Verification items for this drawing (mm, ordinates from the low corner). A direction names the side the tool comes from. Round coordinates to 2 decimals unless told otherwise and drop trailing zeros. Write each loop counter-clockwise with the first axis right and the second up, starting at its lowest first coordinate (ties: lowest second). Pieces come first, ordered by that corner, then holes.
Item 1: Cross-section at D-D (y = 16.5). Enter the section's corners in (x, z).
Item 2: Cross-section at A-A (z = 63.5). Enter the section's corners in (x, y), then the cut area to 3 significant figures.
Item 3: Access from +Z, -Z, +X, -X, +Y, -Y to the whole of each face (thin tool, end or side, straight path). Record for the marked faces 1, 2 and 3.
Item 4: Depth check by flat-ended pin: P1, Ø12.5, axis at x = 110.5, z = 24, coming from the -Y side; P2, Ø15, axis at y = 104.775, z = 22.225, coming from the +X side; P3, Ø6, axis at x = 109, z = 22.5, coming from the +Y side. Enter the tip coordinate at first touch or a pass-through.
Item 5: Draft check along X on the marked faces 4, 5 and 6. Enter one of: pulls with the +X half, pulls with the -X half, needs draft (parallel to the pull), parting line crosses it, or undercut.
Item 6: Scan lines: probe 1 along X at (y, z) = (63.5, 3.75) (3 decimals); probe 2 along Z at (x, y) = (63.5, 2.5); probe 3 along Z at (x, y) = (61.5, 70). Record each from-to range of solid material in increasing order.
Item 7: Cross-section at C-C (y = 63.5). Enter the section's corners in (x, z) (3 decimals), then the cut area to 3 significant figures.
Item 8: Cross-section at B-B (x = 63.5). Enter the section's corners in (y, z), then the cut area to 3 significant figures.
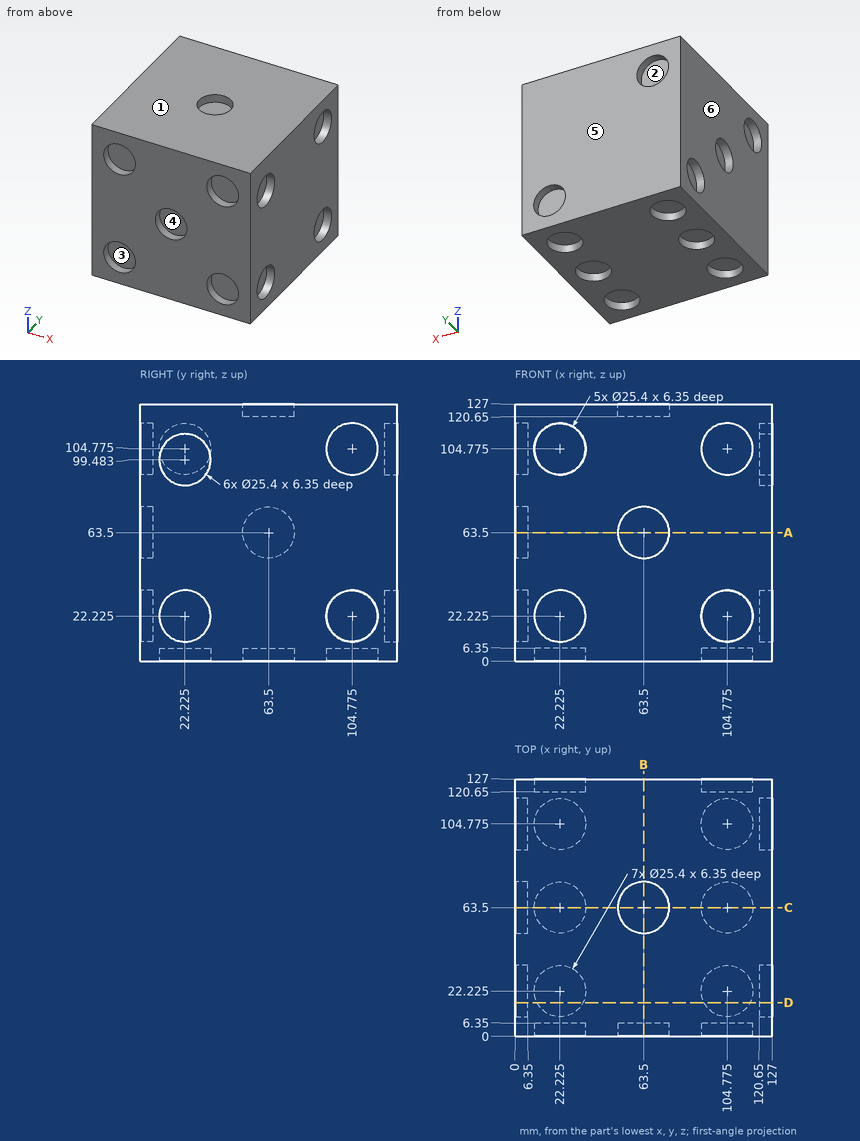
Resolved:
1. outline: (0, 0) - (10.89, 0) - (10.89, 6.35) - (33.56, 6.35) - (33.56, 0) - (93.44, 0) - (93.44, 6.35) - (116.11, 6.35) - (116.11, 0) - (127, 0) - (127, 10.89) - (120.65, 10.89) - (120.65, 33.56) - (127, 33.56) - (127, 88.15) - (120.65, 88.15) - (120.65, 110.82) - (127, 110.82) - (127, 127) - (0, 127) - (0, 116.11) - (6.35, 116.11) - (6.35, 93.44) - (0, 93.44) - close
2. outline: (0, 0) - (50.8, 0) - (50.8, 6.35) - (76.2, 6.35) - (76.2, 0) - (127, 0) - (127, 127) - (0, 127) - (0, 76.2) - (6.35, 76.2) - (6.35, 50.8) - (0, 50.8) - close
2. area: 15,800 mm2
3. face 1: +Z, +X, -X, +Y, -Y
3. face 2: +Y
3. face 3: -Y
4. P1: stops at y = 6.35
4. P2: stops at x = 120.65
4. P3: stops at y = 120.65
5. face 4: undercut
5. face 5: needs draft
5. face 6: pulls with the -X half
6. probe 1: x = 0 to 9.525, 34.925 to 92.075, 117.475 to 127
6. probe 2: z = 0 to 50.8, 76.2 to 127
6. probe 3: z = 0 to 120.65
7. outline: (0, 0) - (9.525, 0) - (9.525, 6.35) - (34.925, 6.35) - (34.925, 0) - (92.075, 0) - (92.075, 6.35) - (117.475, 6.35) - (117.475, 0) - (127, 0) - (127, 127) - (76.2, 127) - (76.2, 120.65) - (50.8, 120.65) - (50.8, 127) - (0, 127) - (0, 76.2) - (6.35, 76.2) - (6.35, 50.8) - (0, 50.8) - close
7. area: 15,500 mm2
8. outline: (0, 0) - (127, 0) - (127, 127) - (76.2, 127) - (76.2, 120.65) - (50.8, 120.65) - (50.8, 127) - (0, 127) - (0, 76.2) - (6.35, 76.2) - (6.35, 50.8) - (0, 50.8) - close
8. area: 15,800 mm2
